from build123d import *

# Parameters (mm, degrees)
SKETCH_1_R      = 6
EXTRUDE_1_DEPTH = 4


# Read off the part's stored shape, not the designer's step: Отверстие обработанное метчиком M31
with BuildPart() as part:
    # Эскиз1 → Бобышка-Вытянуть1 (new, symmetric)
    with BuildSketch(Plane.XY):
        with BuildLine():
            Line((11.124297731, -3.5), (33.5, -3.5))
            Line((33.5, -3.5), (35, -2))
            Line((35, -2), (45, -2))
            Line((45, -2), (45, 2))
            Line((45, 2), (35, 2))
            Line((35, 2), (33.5, 3.5))
            Line((33.5, 3.5), (14.987492178, 3.5))
            ThreePointArc((14.987492178, 3.5), (8.095467802, 6.254311627), (5, 13))
            Line((5, 13), (-5, 13))
            ThreePointArc((-5, 13), (-8.095467802, 6.254311627), (-14.987492178, 3.5))
            Line((-14.987492178, 3.5), (-22.931154754, 3.5))
            ThreePointArc((-22.931154754, 3.5), (-25.707642289, 1.855810024), (-28.910275264, 2.25))
            ThreePointArc((-28.910275264, 2.25), (-32.5, 0), (-28.910275264, -2.25))
            ThreePointArc((-28.910275264, -2.25), (-25.707642289, -1.855810024), (-22.931154754, -3.5))
            Line((-22.931154754, -3.5), (-11.124297731, -3.5))
            ThreePointArc((-11.124297731, -3.5), (-8.90828458, -4.017892715), (-7.151334255, -5.464285714))
            ThreePointArc((-7.151334255, -5.464285714), (0, -9), (7.151334255, -5.464285714))
            ThreePointArc((7.151334255, -5.464285714), (8.90828458, -4.017892715), (11.124297731, -3.5))
        make_face()
        Circle(SKETCH_1_R, mode=Mode.SUBTRACT)
    extrude(amount=EXTRUDE_1_DEPTH, both=True)

    # Отверстие обработанное метчиком M31 outline → Отверстие обработанное метчиком M31 (revolve, cut)
    with BuildSketch(Plane.XY):
        Polygon((0, 5.868327481), (1.25, 5.868327481), (1.25, 12.5), (1.75, 13), (0, 13), align=None)
    revolve(axis=Axis((0, 0, 0), (0, 1, 0)), mode=Mode.SUBTRACT)


solid = part.part
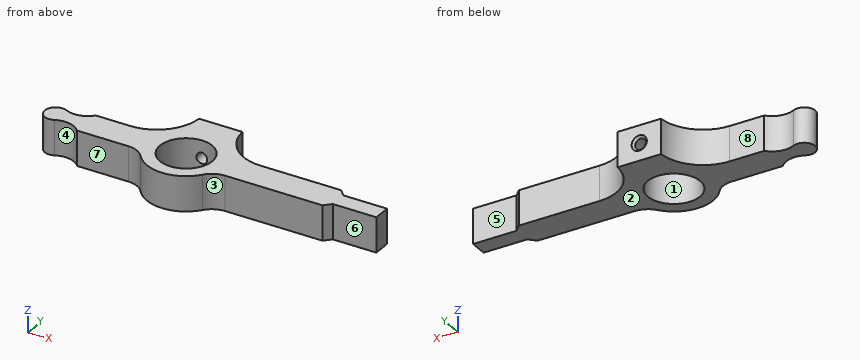
For this review, take the finished solid that the model builds, in its own axes (mm). Face numbers are marked on the shaded views. A direction names the side the tool comes from. Round coordinates to 2 decimals unless told otherwise and drop trailing zeros. Write each loop counter-clockwise with the first axis right and the second up, starting at its lowest first coordinate (ties: lowest second). Pieces come first, ordered by that corner, then holes. Notation, with made-up numbers: (15.5, -38) - (48.5, -38) arc R17 ccw to (48.5, -19) - close; hole circle Ø7 at (-31, 65.25). An arc over 180 degrees is marked (long way). Use a Markdown table: item, result.
Q1. Clearance check with flat-ended pins moving along their axes: pin 1 (2.5 mm diameter, centred on x = -14.5, z = -1, fed in from -Y); pin 2 (3 mm diameter, centred on x = -11, z = 0.5, fed in from -Y); pin 3 (6 mm diameter, centred on x = 15, y = 8.5, fed in from +Z); pin 4 (1 mm diameter, centred on y = 3.5, z = 2.5, fed in from -X). State where each tip first meets the part, or that it passes through.
Derived:
| item | result |
|---|---|
| pin 1 | stops at y = -3.5 |
| pin 2 | stops at y = -3.77 |
| pin 3 | passes through |
| pin 4 | stops at x = -23.42 |
Q2. Wall thickness on line 1 along Z through (x, y) = (0, 8.5); line 2 along Y through (x, z) = (31.5, 1.5); line 3 along Y through (x, z) = (40, 0.25): over which ranges is each line inside the solid? List them lowest first.
Derived:
| item | result |
|---|---|
| line 1 | z = -4 to -1.25, 1.25 to 4 |
| line 2 | y = -3.5 to 3.5 |
| line 3 | y = -2 to 2 |
Q3. Machinability: for the marked faces 5, 6, 7 and 8, which of the approach directions +Z, -Z, +X, -X, +Y, -Y give a long, thin tool a straight path to every point of the face, cutting with its end or side? Answer none if there is none.
Derived:
| item | result |
|---|---|
| face 5 | +Z, -Z, +X, +Y |
| face 6 | +Z, -Z, +X, -Y |
| face 7 | +Z, -Z, -X, -Y |
| face 8 | +Z, -Z, -X, +Y |
Q4. We need section B-B (z = -2.5). Give the boundary of the cut face in (x, y), plus the area to 3 significant figures.
Derived:
| item | result |
|---|---|
| outline | (-28.91, -2.25) arc R5 cw to (-22.93, -3.5) - (-11.12, -3.5) arc R5 cw to (-7.15, -5.46) arc R9 ccw to (7.15, -5.46) arc R5 cw to (11.12, -3.5) - (33.5, -3.5) - (35, -2) - (45, -2) - (45, 2) - (35, 2) - (33.5, 3.5) - (14.99, 3.5) arc R10 cw to (5, 13) - (-5, 13) arc R10 cw to (-14.99, 3.5) - (-22.93, 3.5) arc R5 cw to (-28.91, 2.25) arc R2.5 ccw (long way) to start; hole circle Ø12 at (0, 0) |
| area | 577 mm2 |
Q5. We need section A-A (x = 0). Give the boundary of the cut face in (y, z), plus the area to 4 significant figures.
Derived:
| item | result |
|---|---|
| outline | (-9, -4) - (-6, -4) - (-6, 4) - (-9, 4) - close; (6, -4) - (13, -4) - (13, -1.75) - (12.5, -1.25) - (6, -1.25) - close; (6, 1.25) - (12.5, 1.25) - (13, 1.75) - (13, 4) - (6, 4) - close |
| area | 62.25 mm2 |
Q6. We need section D-D (x = -18). Give the boundary of the cut face in (y, z), plus the area to 3 significant figures.
Derived:
| item | result |
|---|---|
| outline | (-3.5, -4) - (3.5, -4) - (3.5, 4) - (-3.5, 4) - close |
| area | 56.0 mm2 |
Q7. The part is to be moulded in two halves that separate along X. For the marked faces 1, 2, 3 and 4, say which applies: pulls with the +X half, pulls with the -X half, needs draft (parallel to the pull), parting line crosses it, or undercut.
Derived:
| item | result |
|---|---|
| face 1 | undercut |
| face 2 | needs draft |
| face 3 | pulls with the +X half |
| face 4 | undercut |
Q8. We need section C-C (y = 9). Give the boundary of the cut face in (x, z).
Derived:
| item | result |
|---|---|
| outline | (-6.06, -4) - (6.06, -4) - (6.06, 4) - (-6.06, 4) - close; hole circle Ø2.5 at (0, 0) |
